Read the model definition and answer for the solid it produces. Units are mm, in the model's axes. A direction names the side the tool comes from. Coordinates: 2 decimals unless noted, no trailing zeros. Write each loop counter-clockwise with the first axis right and the second up, starting at its lowest first coordinate (ties: lowest second). Pieces come first, ordered by that corner, then holes.
1) The part is cut by section A-A (z = 26.5). Determine the outline of the cut face in (x, y).
2) The part is cut by section C-C (y = 5.5). Determine the outline of the cut face in (x, z), then the cut area to 3 significant figures.
3) Each of these flat-tipped pins is pushed along its axis until it touches: pin 1 Ø4.5 at (x, z) = (0, -28.5) entering from -Y; pin 2 Ø16 at (x, z) = (0, -58.5) entering from -Y. Where does it stop, or does it pass through?
4) Which of the six approach directions +Z, -Z, +X, -X, +Y, -Y give full straight-line access (tool end or side, diameter ignored) to faces 1 (the face through (5.2, 8, -58.7)), 2 (the face through (0.121, 4.93, 23.753))?
5) Determine the mould class of faces 3 (the face through (0, 10, -23)), 4 (the face through (0.484, 4.93, -85.495)), 5 (the face through (0.121, 4.93, -31.247)) for opening direction X: +X half, -X half, draft (parallel to the pull), parting line (faces both ways), or undercut.
6) Find the intervals of material crossed by line 1 (Z direction, x = 2, y = 7.75); line 2 (X direction, y = 1, z = -58); line 3 (X direction, y = 7, z = 26.5), in increasing order.
7) The part is cut by section B-B (x = 0). Determine the outline of the cut face in (y, z), then the cut area to 3 significant figures.
8) The part is cut by section D-D (z = -58.5). Determine the outline of the cut face in (x, y).
from build123d import *

# Parameters (mm, degrees)
SKETCH1_R           = 2.75
SKETCH1_R_2         = 12.1
BOSS_EXTRUDE1_DEPTH = 8
SKETCH2_R           = 2.75
SKETCH2_R_2         = 5
BOSS_EXTRUDE2_DEPTH = 2


with BuildPart() as part:
    # Sketch1 → Boss-Extrude1 (new body)
    with BuildSketch(Plane(origin=(0, 0, 0), x_dir=(1, 0, 0), z_dir=(0, 1, 0))):
        with BuildLine():
            Line((-22, 63.5), (-22, 41.5))
            Line((-22, 41.5), (-22, -41.5))
            Line((-22, -41.5), (22, -41.5))
            Line((22, -41.5), (22, 41.5))
            Line((22, 41.5), (22, 63.5))
            ThreePointArc((22, 63.5), (0, 85.5), (-22, 63.5))
        make_face()
        with Locations(Location((0, -26.5, 0), (0, 0, 270))):
            Circle(SKETCH1_R, mode=Mode.SUBTRACT)
        with Locations(Location((0, 58.5, 0), (0, 0, 270))):
            Circle(SKETCH1_R_2, mode=Mode.SUBTRACT)
        with Locations(Location((0, 28.5, 0), (0, 0, 270))):
            Circle(SKETCH1_R, mode=Mode.SUBTRACT)
    extrude(amount=BOSS_EXTRUDE1_DEPTH)

    # Sketch2 → Boss-Extrude2 (add)
    with BuildSketch(Plane(origin=(0, 8, 0), x_dir=(1, 0, 0), z_dir=(0, 1, 0))):
        with BuildLine():
            Line((-22, -41.5), (22, -41.5))
            Line((22, -41.5), (22, 63.5))
            ThreePointArc((22, 63.5), (0, 85.5), (-22, 63.5))
            Line((-22, 63.5), (-22, -41.5))
        make_face()
        with Locations(Location((0, 28.5, 0), (0, 0, 270))):
            Circle(SKETCH2_R, mode=Mode.SUBTRACT)
        with Locations(Location((0, -26.5, 0), (0, 0, 270))):
            Circle(SKETCH2_R, mode=Mode.SUBTRACT)
        with Locations(Location((0, 58.5, 0), (0, 0, 270))):
            Circle(SKETCH2_R_2, mode=Mode.SUBTRACT)
    extrude(amount=BOSS_EXTRUDE2_DEPTH)


solid = part.part
Reported:
1. outline: (-22, 0) - (-2.75, 0) - (-2.75, 10) - (-22, 10) - close; (2.75, 0) - (22, 0) - (22, 10) - (2.75, 10) - close
2. outline: (-22, -63.5) arc R22 ccw to (22, -63.5) - (22, 41.5) - (-22, 41.5) - close; hole circle Ø24.2 at (0, -58.5); hole circle Ø5.5 at (0, -28.5); hole circle Ø5.5 at (0, 26.5)
2. area: 4,870 mm2
3. pin 1: passes through
3. pin 2: stops at y = 8
4. face 1: -Y
4. face 2: +Y, -Y
5. face 3: draft
5. face 4: parting line
5. face 5: undercut
6. line 1: z = -85.41 to -70.43, -46.57 to -30.39, -26.61 to 24.61, 28.39 to 41.5
6. line 2: x = -22 to -12.09, 12.09 to 22
6. line 3: x = -22 to -2.75, 2.75 to 22
7. outline: (0, -85.5) - (10, -85.5) - (10, -63.5) - (8, -63.5) - (8, -70.6) - (0, -70.6) - close; (0, -46.4) - (8, -46.4) - (8, -53.5) - (10, -53.5) - (10, -31.25) - (0, -31.25) - close; (0, -25.75) - (10, -25.75) - (10, 23.75) - (0, 23.75) - close; (0, 29.25) - (10, 29.25) - (10, 41.5) - (0, 41.5) - close
7. area: 946 mm2
8. outline: (-22, 0) - (-12.1, 0) - (-12.1, 8) - (-5, 8) - (-5, 10) - (-22, 10) - close; (5, 8) - (12.1, 8) - (12.1, 0) - (22, 0) - (22, 10) - (5, 10) - close
